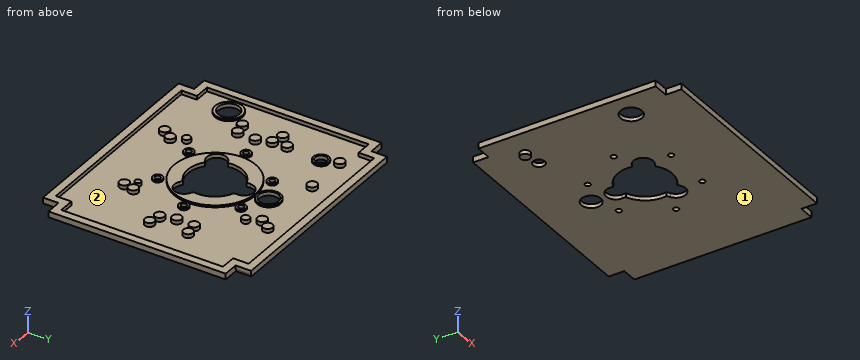
```python
from build123d import *

# Parameters (mm, degrees)
F1_DEPTH  = 5
F3_DEPTH  = 10
F4_R      = 20
F4_R_2    = 30
F4_R_3    = 105
F4_R_4    = 12.5
F4_R_5    = 35
F5_DEPTH  = 5
F6_R      = 27.5
F6_R_2    = 7
F6_R_3    = 25
F6_R_4    = 15
F7_DEPTH  = 10
F8_R      = 12.5
F8_R_2    = 10
F8_R_3    = 7.5
F9_DEPTH  = 10
F10_R     = 12.5
F11_DEPTH = 10


with BuildPart() as f1:
    # F0 (on Top) → F1 (new body)
    with BuildSketch(Plane.XY):
        Polygon((-270, -228), (-270, -268), (270, -268), (270, -228), (310, -228), (310, 228), (270, 228), (270, 268), (-270, 268), (-270, 228), (-310, 228), (-310, -228), align=None)
    extrude(amount=F1_DEPTH)

    # F2 (on face) → F3 (join)
    with BuildSketch(Plane.XY.offset(5)):
        Polygon((-270, -228), (-270, -268), (270, -268), (270, -228), (310, -228), (310, 228), (270.789407, 228), (270.789407, 268), (-270, 268), (-270, 228), (-310, 228), (-310, -228), align=None)
        Polygon((250, 248), (250, 208), (290, 208), (290, -208), (250, -208), (250, -248), (-250, -248), (-250, -208), (-290, -208), (-290, 208), (-250, 208), (-250, 248), align=None, mode=Mode.SUBTRACT)
    extrude(amount=F3_DEPTH)

    # F4 (on face) → F5 (join)
    with BuildSketch(Plane.XY.offset(5)):
        with Locations((-190, 150)):
            Circle(F4_R)
        with Locations((0, 138.5)):
            Circle(F4_R_2)
        Circle(F4_R_3)
        with Locations((-124, 0)):
            Circle(F4_R_4)
        with Locations((-245, -123)):
            Circle(F4_R_5)
        with Locations((-62, 107.38715)):
            Circle(F4_R_4)
        with Locations((62, 107.38715)):
            Circle(F4_R_4)
        with Locations((124, 0)):
            Circle(F4_R_4)
        with Locations((62, -107.38715)):
            Circle(F4_R_4)
        with Locations((-62, -107.38715)):
            Circle(F4_R_4)
    extrude(amount=F5_DEPTH)

    # F6 (on face) → F7 (cut, through all)
    with BuildSketch(Plane.XY.offset(10)):
        with Locations((-245, -123)):
            Circle(F6_R)
        with Locations((-124, 0)):
            Circle(F6_R_2)
        with Locations((0, 138.5)):
            Circle(F6_R_3)
        with Locations((-190, 150)):
            Circle(F6_R_4)
        with Locations((-62, -107.38715)):
            Circle(F6_R_2)
        with Locations((62, -107.38715)):
            Circle(F6_R_2)
        with Locations((124, 0)):
            Circle(F6_R_2)
        with Locations((62, 107.38715)):
            Circle(F6_R_2)
        with Locations((-62, 107.38715)):
            Circle(F6_R_2)
        with BuildLine():
            Line((25, 65.383484), (25, 75))
            ThreePointArc((25, 75), (0, 100), (-25, 75))
            Line((-25, 75), (-25, 65.383484))
            ThreePointArc((-25, 65.383484), (-60.621778, 35), (-69.123758, -11.041107))
            Line((-69.123758, -11.041107), (-77.451905, -15.849365))
            ThreePointArc((-77.451905, -15.849365), (-86.60254, -50), (-52.451905, -59.150635))
            Line((-52.451905, -59.150635), (-44.123758, -54.342377))
            ThreePointArc((-44.123758, -54.342377), (0, -70), (44.123758, -54.342377))
            Line((44.123758, -54.342377), (52.451905, -59.150635))
            ThreePointArc((52.451905, -59.150635), (86.60254, -50), (77.451905, -15.849365))
            Line((77.451905, -15.849365), (69.123758, -11.041107))
            ThreePointArc((69.123758, -11.041107), (60.621778, 35), (25, 65.383484))
        make_face()
    extrude(amount=-F7_DEPTH, mode=Mode.SUBTRACT)

    # F8 (on face) → F9 (join)
    with BuildSketch(Plane.XY.offset(5)):
        with Locations((-101, -195)):
            Circle(F8_R)
        with Locations((-84, -170)):
            Circle(F8_R)
        with Locations((-179, -12)):
            Circle(F8_R)
        with Locations((-211, -66)):
            Circle(F8_R)
        with Locations((-182, -59)):
            Circle(F8_R)
        with Locations((-220, 32)):
            Circle(F8_R)
        with Locations((-191, 24)):
            Circle(F8_R)
        with Locations((-192.5, 61)):
            Circle(F8_R)
        with Locations((-200, 192)):
            Circle(F8_R)
        with Locations((-90, 192)):
            Circle(F8_R)
        with Locations((84, 176)):
            Circle(F8_R)
        with Locations((101, 201)):
            Circle(F8_R)
        with Locations((182, 64)):
            Circle(F8_R)
        with Locations((212, 68)):
            Circle(F8_R)
        with Locations((179.5, 18)):
            Circle(F8_R)
        with Locations((191, -19)):
            Circle(F8_R)
        with Locations((220, -26)):
            Circle(F8_R)
        with Locations((124, -153)):
            Circle(F8_R)
        with Locations((130, -126)):
            Circle(F8_R)
        with Locations((-99, -137)):
            Circle(F8_R_2)
        with Locations((99, 143)):
            Circle(F8_R_2)
        with Locations((104, -131)):
            Circle(F8_R_3)
    extrude(amount=F9_DEPTH)

    # F10 (on face) → F11 (join)
    with BuildSketch(Plane(origin=(0, 0, 0), x_dir=(1, 0, 0), z_dir=(0, 0, -1))):
        with Locations((-240, -153)):
            Circle(F10_R)
    extrude(amount=F11_DEPTH)


solid = f1.part
```
CAD build for the part. Positions are in the model's coordinates, mm. Face numbers are marked on the shaded views. Coordinates: 2 decimals unless noted, no trailing zeros. Order: outer loops, then holes, each group sorted by start corner. A loop starts at its lowest first (then second) coordinate and runs counter-clockwise, first axis right, second up. Notation, with made-up numbers: M -21.5,-19.5 L 10.5,-19.5 A24 cw 10.5,12.5 Z; hole C -4.5,15.5 d9. An arc over 180 degrees is marked long. Write each question's results on one line, items separated by ' | '. Start each with the question number.
Q1. Drill centre lines: probe 1 along Y at (x, z) = (-124, 5.5); probe 2 along Y at (x, z) = (-2.5, 9.5); probe 3 along X at (y, z) = (-35, 3). Where is each one in solid material? Low to high. Write a range as from..to.
Q2. Pull direction X, two halves, no side cores. Call the marked faces 1 and 2: +X half, -X half, draft (parallel to the pull), parting line (faces both ways), or undercut.
Q3. Cut at B-B (z = -4.75). List the corners of the cut face in (x, y), then the cut area to 3 significant figures.
Q4. Cut at A-A (x = 62). Count the separate pieces of the cut face and the enclosed holes in it, then the cut area to 3 significant figures.
Q5. Flat gauge pins, fed straight in: P1, Ø12, axis at x = 281, z = 10, coming from the -Y side; P2, Ø8, axis at x = 45.5, y = -202, coming from the +Z side; P3, Ø4.5, axis at y = -242, z = 6.5, coming from the -X side; P4, Ø11, axis at x = 62, y = -107.39, coming from the +Z side. Where does each tip first touch, or does it go through?
Found:
1) probe 1: -268..-248, -12.5..-7, 7..12.5, 248..268 | probe 2: -268..-248, -104.97..-69.96, 99.87..104.97, 108.6..113.63, 163.37..168.4, 248..268 | probe 3: -310..-89.83, 89.83..310
2) face 1: draft | face 2: undercut
3) outline: C -240,153 d25 | area: 491 mm²
4) separate pieces: 4 | enclosed holes: 0 | area: 2,950 mm²
5) P1: y = -228 | P2: z = 5 | P3: x = -270 | P4: through
